Check sheet for the modelled part. Datum: model origin and axes. Units: mm. Face numbers are marked on the shaded views. A direction names the side the tool comes from. Round coordinates to 2 decimals unless told otherwise and drop trailing zeros. Write each loop counter-clockwise with the first axis right and the second up, starting at its lowest first coordinate (ties: lowest second). Pieces come first, ordered by that corner, then holes.
Item 1: Release check for a two-part mould opening along Y. For the marked faces 6, 7, 8 and 9 record: +Y half, -Y half, draft (parallel to the pull), parting line (faces both ways), or undercut.
Item 2: Cross-section at A-A on y = 52. Enter the section's corners in (x, z).
Item 3: Tool access check on the marked faces 1, 2, 3, 4 and 5. Record the directions out of +Z, -Z, +X, -X, +Y, -Y that give a thin tool (end or side, any length) a straight path to the whole face; none if there is none.
Item 4: Cross-section at B-B on z = 7. Count the separate pieces of the cut face and the enclosed holes in it, plus the area to 3 significant figures.
Item 5: Material ranges on line 1 (Y direction, x = -16, z = 2); line 2 (Z direction, x = 17, y = 53.5); line 3 (Y direction, x = -10, z = -5.5), recorded low to high.
Item 6: Go/stop test with flat-tipped pins: pin 1 Ø8.5 at (y, z) = (14, -18) entering from -X; pin 2 Ø3 at (x, z) = (-1.5, 9.5) entering from -Y; pin 3 Ø2.5 at (y, z) = (15, -5.5) entering from -X; pin 4 Ø4 at (y, z) = (51, 23.5) entering from -X. Record where each tip stops, or that it passes through.
from build123d import *

# Parameters (mm, degrees)
EXTRUDE_5_DEPTH      = 66
CUT_EXTRUDE_1_DEPTH  = 83.95179323
SKETCH_6_4_R         = 2.5
CUT_EXTRUDE_3_DEPTH  = 83.95179323
CUT_EXTRUDE_5_DEPTH  = 83.95179323
EXTRUDE_9_DEPTH      = 4
SKETCH_16_R          = 2.5
CUT_EXTRUDE_6_DEPTH  = 81.950602221
SKETCH_21_R          = 2.5
CUT_EXTRUDE_9_DEPTH  = 79.193669821
CUT_EXTRUDE_10_DEPTH = 4.7
EXTRUDE_START        = -9
SKETCH_26_R          = 2.5
EXTRUDE_11_DEPTH     = 9
SKETCH_27_R          = 2.5
EXTRUDE_12_DEPTH     = 9
SKETCH_25_R          = 1.5
CUT_EXTRUDE_12_DEPTH = 10
SKETCH_30_W          = 2.5
SKETCH_30_H          = 5.5
CUT_EXTRUDE_13_DEPTH = 8
SKETCH_31_R          = 2.6
CUT_EXTRUDE_14_DEPTH = 83.95179323
CUT_EXTRUDE_15_DEPTH = 39
SKETCH_33_R          = 2.6
CUT_EXTRUDE_16_DEPTH = 79.193669821
CUT_EXTRUDE_17_DEPTH = 4.7
SKETCH_35_R          = 10.75
CUT_EXTRUDE_18_DEPTH = 75.123208241
SKETCH_36_W          = 3.5
SKETCH_36_H          = 7
SKETCH_36_W_2        = 2.5
SKETCH_36_H_2        = 5.5
CUT_EXTRUDE_19_DEPTH = 7.5
SKETCH_37_R          = 1.7
CUT_EXTRUDE_20_DEPTH = 14


with BuildPart() as part:
    # Эскиз1 → Бобышка-Вытянуть5 (new body)
    with BuildSketch(Plane(origin=(0, 0, 0), x_dir=(1, 0, 0), z_dir=(0, 1, 0))):
        with BuildLine():
            Line((-21.5, 10), (-21.5, 1))
            Line((-21.5, 1), (-5.45227248, 1))
            ThreePointArc((-5.45227248, 1), (15.5, 0), (-5.45227248, -1))
            Line((-5.45227248, -1), (-21.5, -1))
            Line((-21.5, -1), (-21.5, -10))
            Line((-21.5, -10), (-10.5, -10))
            Line((-10.5, -10), (-1.750859731, -18))
            Line((-1.750859731, -18), (13.5, -18))
            Line((13.5, -18), (13.5, -26))
            Line((13.5, -26), (21.5, -26))
            Line((21.5, -26), (21.5, -18))
            Line((21.5, -18), (21.5, 18))
            Line((21.5, 18), (21.5, 26))
            Line((21.5, 26), (13.5, 26))
            Line((13.5, 26), (13.5, 18))
            Line((13.5, 18), (-1.750859731, 18))
            Line((-1.750859731, 18), (-10.5, 10))
            Line((-10.5, 10), (-21.5, 10))
        make_face()
    extrude(amount=EXTRUDE_5_DEPTH)

    # Эскиз6 → Вырез-Вытянуть1 (cut, through all)
    with BuildSketch(Plane(origin=(21.5, 0, 0), x_dir=(0, 0, -1), z_dir=(1, 0, 0))):
        Polygon((-18, 61.237604307), (-18, 66), (-26, 66), (-26, 56.618802154), align=None)
        Polygon((-18, 42.762395693), (-26, 47.381197846), (-26, 37.618802154), (-18, 42.237604307), align=None)
        Polygon((-18, 23.762395693), (-26, 28.381197846), (-26, 18.618802154), (-18, 23.237604307), align=None)
        Polygon((-18, 4.762395693), (-26, 9.381197846), (-26, 0.083563763), (-26, 0), (-18, 0), align=None)
        Polygon((26, 0), (26, 9.381197846), (18, 4.762395693), (18, 0), align=None)
        Polygon((26, 18.618802154), (26, 28.381197846), (18, 23.762395693), (18, 23.237604307), align=None)
        Polygon((26, 37.618802154), (26, 47.381197846), (18, 42.762395693), (18, 42.237604307), align=None)
        Polygon((26, 66), (18, 66), (18, 61.237604307), (26, 56.618802154), align=None)
    extrude(amount=-CUT_EXTRUDE_1_DEPTH, mode=Mode.SUBTRACT)

    # Эскиз6<4> → Вырез-Вытянуть3 (cut, through all)
    with BuildSketch(Plane(origin=(21.5, 0, 0), x_dir=(0, 0, -1), z_dir=(1, 0, 0))):
        with Locations((-18, 52)):
            Circle(SKETCH_6_4_R)
        with Locations((-18, 33)):
            Circle(SKETCH_6_4_R)
        with Locations((-18, 14)):
            Circle(SKETCH_6_4_R)
        with Locations((18, 14)):
            Circle(SKETCH_6_4_R)
        with Locations((18, 33)):
            Circle(SKETCH_6_4_R)
        with Locations((18, 52)):
            Circle(SKETCH_6_4_R)
    extrude(amount=-CUT_EXTRUDE_3_DEPTH, mode=Mode.SUBTRACT)

    # Эскиз10 → Вырез-Вытянуть5 (cut, through all)
    with BuildSketch(Plane(origin=(21.5, 0, 0), x_dir=(0, 0, -1), z_dir=(1, 0, 0))):
        Polygon((14, 16.309401077), (14, 11.690598923), (18, 9.381197846), (22, 11.690598923), (22, 16.309401077), (18, 18.618802154), align=None)
        Polygon((14, 35.309401077), (14, 30.690598923), (18, 28.381197846), (22, 30.690598923), (22, 35.309401077), (18, 37.618802154), align=None)
        Polygon((14, 54.309401077), (14, 49.690598923), (18, 47.381197846), (22, 49.690598923), (22, 54.309401077), (18, 56.618802154), align=None)
        Polygon((-18, 56.618802154), (-14, 54.309401077), (-14, 49.690598923), (-18, 47.381197846), (-22, 49.690598923), (-22, 54.309401077), align=None)
        Polygon((-18, 37.618802154), (-14, 35.309401077), (-14, 30.690598923), (-18, 28.381197846), (-22, 30.690598923), (-22, 35.309401077), align=None)
        Polygon((-18, 18.618802154), (-14, 16.309401077), (-14, 11.690598923), (-18, 9.381197846), (-22, 11.690598923), (-22, 16.309401077), align=None)
    extrude(amount=-CUT_EXTRUDE_5_DEPTH, mode=Mode.SUBTRACT)

    # Эскиз12 → Бобышка-Вытянуть9 (add)
    with BuildSketch(Plane(origin=(21.5, 0, 0), x_dir=(0, 0, -1), z_dir=(1, 0, 0))):
        Polygon((-14, 49.690598923), (-14, 54.309401077), (-18, 56.618802154), (-22, 54.309401077), (-22, 49.690598923), (-18, 47.381197846), align=None)
        Polygon((-14, 30.690598923), (-14, 35.309401077), (-18, 37.618802154), (-22, 35.309401077), (-22, 30.690598923), (-18, 28.381197846), align=None)
        Polygon((-14, 11.690598923), (-14, 16.309401077), (-18, 18.618802154), (-22, 16.309401077), (-22, 11.690598923), (-18, 9.381197846), align=None)
        Polygon((22, 49.690598923), (22, 54.309401077), (18, 56.618802154), (14, 54.309401077), (14, 49.690598923), (18, 47.381197846), align=None)
        Polygon((22, 30.690598923), (22, 35.309401077), (18, 37.618802154), (14, 35.309401077), (14, 30.690598923), (18, 28.381197846), align=None)
        Polygon((22, 11.690598923), (22, 16.309401077), (18, 18.618802154), (14, 16.309401077), (14, 11.690598923), (18, 9.381197846), align=None)
    extrude(amount=-EXTRUDE_9_DEPTH)

    # Эскиз16 → Вырез-Вытянуть6 (cut, through all)
    with BuildSketch(Plane.ZY.offset(-17.5)):
        with Locations((-18, 52)):
            Circle(SKETCH_16_R)
        with Locations((-18, 33)):
            Circle(SKETCH_16_R)
        with Locations((-18, 14)):
            Circle(SKETCH_16_R)
        with Locations((18, 14)):
            Circle(SKETCH_16_R)
        with Locations((18, 33)):
            Circle(SKETCH_16_R)
        with Locations((18, 52)):
            Circle(SKETCH_16_R)
    extrude(amount=-CUT_EXTRUDE_6_DEPTH, mode=Mode.SUBTRACT)

    # Эскиз21 → Вырез-Вытянуть9 (cut, through all)
    with BuildSketch(Plane.XY.offset(10)):
        with Locations(Location((-16, 59, 0), (0, 0, 180))):
            Circle(SKETCH_21_R)
        with Locations(Location((-16, 43, 0), (0, 0, 180))):
            Circle(SKETCH_21_R)
        with Locations(Location((-16, 23, 0), (0, 0, 180))):
            Circle(SKETCH_21_R)
        with Locations(Location((-16, 7, 0), (0, 0, 180))):
            Circle(SKETCH_21_R)
        with Locations(Location((-16, 33, 0), (0, 0, 180))):
            Circle(SKETCH_21_R)
    extrude(amount=-CUT_EXTRUDE_9_DEPTH, mode=Mode.SUBTRACT)

    # Эскиз22 → Вырез-Вытянуть10 (cut)
    with BuildSketch(Plane.XY.offset(10)):
        Polygon((-12, 56.690598923), (-12, 61.309401077), (-16, 63.618802154), (-20, 61.309401077), (-20, 56.690598923), (-16, 54.381197846), align=None)
        Polygon((-12, 40.690598923), (-12, 45.309401077), (-16, 47.618802154), (-20, 45.309401077), (-20, 40.690598923), (-16, 38.381197846), align=None)
        Polygon((-16, 27.618802154), (-12, 25.309401077), (-12, 20.690598923), (-16, 18.381197846), (-20, 20.690598923), (-20, 25.309401077), align=None)
        Polygon((-16, 11.618802154), (-12, 9.309401077), (-12, 4.690598923), (-16, 2.381197846), (-20, 4.690598923), (-20, 9.309401077), align=None)
    extrude(amount=-CUT_EXTRUDE_10_DEPTH, mode=Mode.SUBTRACT)

    # Эскиз26 → Бобышка-Вытянуть11 (add)
    with BuildSketch(Plane(origin=(0, 0, -10), x_dir=(-1, 0, 0), z_dir=(0, 0, -1)).offset(EXTRUDE_START)):
        with Locations(Location((16, 33, 0), (0, 0, 180))):
            Circle(SKETCH_26_R)
    extrude(amount=EXTRUDE_11_DEPTH)

    # Эскиз27 → Бобышка-Вытянуть12 (add)
    with BuildSketch(Plane.XY.offset(10)):
        with Locations((-16, 33)):
            Circle(SKETCH_27_R)
    extrude(amount=-EXTRUDE_12_DEPTH)

    # Эскиз25 → Вырез-Вытянуть12 (cut)
    with BuildSketch(Plane.ZY.offset(21.5)):
        with Locations((-5.5, 15)):
            Circle(SKETCH_25_R)
        with Locations((-5.5, 33)):
            Circle(SKETCH_25_R)
    extrude(amount=-CUT_EXTRUDE_12_DEPTH, mode=Mode.SUBTRACT)

    # Эскиз30 → Вырез-Вытянуть13 (cut)
    with BuildSketch(Plane(origin=(0, 0, -10), x_dir=(-1, 0, 0), z_dir=(0, 0, -1))):
        with Locations((16, 33)):
            Rectangle(SKETCH_30_W, SKETCH_30_H)
        with Locations((16, 15)):
            Rectangle(SKETCH_30_W, SKETCH_30_H)
    extrude(amount=-CUT_EXTRUDE_13_DEPTH, mode=Mode.SUBTRACT)

    # Эскиз31 → Вырез-Вытянуть14 (cut, through all)
    with BuildSketch(Plane(origin=(21.5, 0, 0), x_dir=(0, 0, -1), z_dir=(1, 0, 0))):
        with Locations((18, 52)):
            Circle(SKETCH_31_R)
        with Locations((18, 33)):
            Circle(SKETCH_31_R)
        with Locations((18, 14)):
            Circle(SKETCH_31_R)
        with Locations((-18, 14)):
            Circle(SKETCH_31_R)
        with Locations((-18, 33)):
            Circle(SKETCH_31_R)
        with Locations((-18, 52)):
            Circle(SKETCH_31_R)
    extrude(amount=-CUT_EXTRUDE_14_DEPTH, mode=Mode.SUBTRACT)

    # Эскиз32 → Вырез-Вытянуть15 (cut)
    with BuildSketch(Plane.ZY.offset(21.5)):
        Polygon((18, 28.265727793), (22.1, 30.632863896), (22.1, 35.367136104), (18, 37.734272207), (13.9, 35.367136104), (13.9, 30.632863896), align=None)
        Polygon((18, 9.265727793), (22.1, 11.632863896), (22.1, 16.367136104), (18, 18.734272207), (13.9, 16.367136104), (13.9, 11.632863896), align=None)
        Polygon((-18, 9.265727793), (-13.9, 11.632863896), (-13.9, 16.367136104), (-18, 18.734272207), (-22.1, 16.367136104), (-22.1, 11.632863896), align=None)
        Polygon((-18, 28.265727793), (-13.9, 30.632863896), (-13.9, 35.367136104), (-18, 37.734272207), (-22.1, 35.367136104), (-22.1, 30.632863896), align=None)
        Polygon((-18, 47.265727793), (-13.9, 49.632863896), (-13.9, 54.367136104), (-18, 56.734272207), (-22.1, 54.367136104), (-22.1, 49.632863896), align=None)
        Polygon((18, 47.265727793), (22.1, 49.632863896), (22.1, 54.367136104), (18, 56.734272207), (13.9, 54.367136104), (13.9, 49.632863896), align=None)
    extrude(amount=-CUT_EXTRUDE_15_DEPTH, mode=Mode.SUBTRACT)

    # Эскиз33 → Вырез-Вытянуть16 (cut, through all)
    with BuildSketch(Plane.XY.offset(10)):
        with Locations((-16, 59)):
            Circle(SKETCH_33_R)
        with Locations((-16, 43)):
            Circle(SKETCH_33_R)
        with Locations(Location((-16, 23, 0), (0, 0, 180))):
            Circle(SKETCH_33_R)
        with Locations(Location((-16, 7, 0), (0, 0, 180))):
            Circle(SKETCH_33_R)
    extrude(amount=-CUT_EXTRUDE_16_DEPTH, mode=Mode.SUBTRACT)

    # Эскиз34 → Вырез-Вытянуть17 (cut)
    with BuildSketch(Plane.XY.offset(10)):
        Polygon((-16, 54.265727793), (-11.9, 56.632863896), (-11.9, 61.367136104), (-16, 63.734272207), (-20.1, 61.367136104), (-20.1, 56.632863896), align=None)
        Polygon((-16, 38.265727793), (-11.9, 40.632863896), (-11.9, 45.367136104), (-16, 47.734272207), (-20.1, 45.367136104), (-20.1, 40.632863896), align=None)
        Polygon((-16, 18.265727793), (-11.9, 20.632863896), (-11.9, 25.367136104), (-16, 27.734272207), (-20.1, 25.367136104), (-20.1, 20.632863896), align=None)
        Polygon((-16, 2.265727793), (-11.9, 4.632863896), (-11.9, 9.367136104), (-16, 11.734272207), (-20.1, 9.367136104), (-20.1, 4.632863896), align=None)
    extrude(amount=-CUT_EXTRUDE_17_DEPTH, mode=Mode.SUBTRACT)

    # Эскиз35 → Вырез-Вытянуть18 (cut, through all)
    with BuildSketch(Plane.XZ):
        with Locations((5, 0)):
            Circle(SKETCH_35_R)
    extrude(amount=-CUT_EXTRUDE_18_DEPTH, mode=Mode.SUBTRACT)

    # Эскиз36 → Вырез-Вытянуть19 (cut)
    # profile 1 of 3: a face of its own
    with BuildSketch(Plane(origin=(0, 0, -10), x_dir=(-1, 0, 0), z_dir=(0, 0, -1))):
        with Locations((16, 15)):
            Rectangle(SKETCH_36_W, SKETCH_36_H)
        with Locations((16, 15)):
            Rectangle(SKETCH_36_W_2, SKETCH_36_H_2, mode=Mode.SUBTRACT)
    # profile 2 of 3: a face of its own
    with BuildSketch(Plane(origin=(0, 0, -10), x_dir=(-1, 0, 0), z_dir=(0, 0, -1))):
        with Locations((16, 15)):
            Rectangle(SKETCH_36_W_2, SKETCH_36_H_2)
    # profile 3 of 3: a face of its own
    with BuildSketch(Plane(origin=(0, 0, -10), x_dir=(-1, 0, 0), z_dir=(0, 0, -1))):
        with Locations((16, 33)):
            Rectangle(SKETCH_36_W, SKETCH_36_H)
    extrude(amount=-CUT_EXTRUDE_19_DEPTH, mode=Mode.SUBTRACT)

    # Эскиз37 → Вырез-Вытянуть20 (cut)
    with BuildSketch(Plane.ZY.offset(21.5)):
        with Locations((-5.5, 33)):
            Circle(SKETCH_37_R)
        with Locations((-5.5, 15)):
            Circle(SKETCH_37_R)
    extrude(amount=-CUT_EXTRUDE_20_DEPTH, mode=Mode.SUBTRACT)


solid = part.part
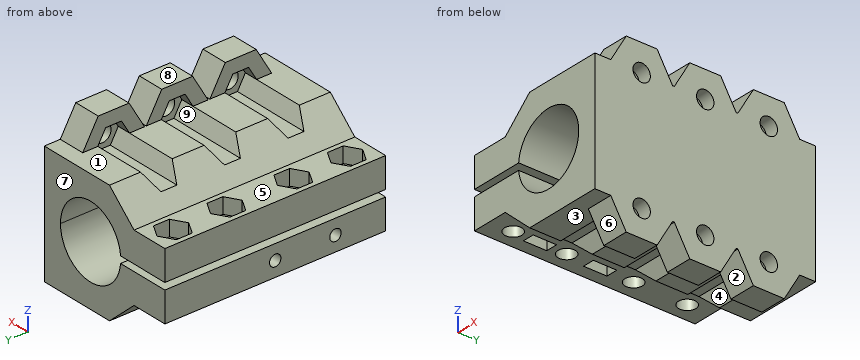
Response values:
1. face 6: -Y half
1. face 7: +Y half
1. face 8: draft
1. face 9: undercut
2. outline: (-21.5, -10) - (-10.5, -10) - (-6.23, -13.9) - (17.5, -13.9) - (17.5, -15.4) - (21.5, -15.4) - (21.5, 15.4) - (17.5, 15.4) - (17.5, 13.9) - (-6.23, 13.9) - (-10.5, 10) - (-21.5, 10) - (-21.5, 1) - (-5.7, 1) arc R10.75 cw (long way) to (-5.7, -1) - (-21.5, -1) - close; (13.5, -26) - (21.5, -26) - (21.5, -20.6) - (17.5, -20.6) - (17.5, -22.1) - (13.5, -22.1) - close; (13.5, 22.1) - (17.5, 22.1) - (17.5, 20.6) - (21.5, 20.6) - (21.5, 26) - (13.5, 26) - close
3. face 1: +Z, -X, +Y
3. face 2: -Z, +X, -X
3. face 3: -Z, -X, -Y
3. face 4: -X
3. face 5: +Z, -X, +Y, -Y
4. separate pieces: 2
4. enclosed holes: 4
4. area: 1,530 mm2
5. line 1: y = 0 to 4.4, 9.6 to 20.4, 25.6 to 40.4, 45.6 to 56.4, 61.6 to 66
5. line 2: z = -26 to -22.1, -13.9 to 13.9, 22.1 to 26
5. line 3: y = 0 to 13.3, 16.7 to 31.3, 34.7 to 66
6. pin 1: stops at x = -6.4
6. pin 2: stops at y = 0
6. pin 3: stops at x = -7.5
6. pin 4: stops at x = 13.5
